Read the model definition and answer for the solid it produces. Units are mm, in the model's axes. A direction names the side the tool comes from. Round coordinates to 2 decimals unless told otherwise and drop trailing zeros. Order: outer loops, then holes, each group sorted by start corner. A loop starts at its lowest first (then second) coordinate and runs counter-clockwise, first axis right, second up.
from build123d import *

# Parameters (mm, degrees)
BOSS_EXTRUDE1_DEPTH  = 10.16
SKETCH2_R            = 2.032
BOSS_EXTRUDE2_DEPTH  = 3.302
SKETCH3_W            = 1.778
SKETCH3_H            = 8.255
BOSS_EXTRUDE3_DEPTH  = 12.7
SKETCH4_W            = 1.524
SKETCH4_H            = 8.255
BOSS_EXTRUDE4_DEPTH  = 2.286
BOSS_EXTRUDE5_DEPTH  = 2.54
BOSS_EXTRUDE6_DEPTH  = 3.556
SKETCH7_W            = 2.032
SKETCH7_H            = 8.255
BOSS_EXTRUDE7_DEPTH  = 2.032
SKETCH8_W            = 1.524
SKETCH8_H            = 8.255
BOSS_EXTRUDE8_DEPTH  = 4.826
SKETCH9_W            = 1.524
SKETCH9_H            = 22.86
BOSS_EXTRUDE9_DEPTH  = 0.254
FILLET2_R            = 0.254
FILLET4_R            = 0.254
FILLET2_OF_MIRROR1_R = 0.254
FILLET4_OF_MIRROR1_R = 0.254
SKETCH10_R           = 3.7084
CUT_EXTRUDE1_DEPTH   = 1.27


with BuildPart() as part:
    # Sketch1 → Boss-Extrude1 (new body)
    with BuildSketch(Plane(origin=(0, 0, 0), x_dir=(1, 0, 0), z_dir=(0, 1, 0))):
        with BuildLine():
            Line((-64.135, 14.859), (64.135, 14.859))
            ThreePointArc((64.135, 14.859), (65.931051224, 14.115051224), (66.675, 12.319))
            Line((66.675, 12.319), (66.675, -12.319))
            ThreePointArc((66.675, -12.319), (65.931051224, -14.115051224), (64.135, -14.859))
            Line((64.135, -14.859), (-64.135, -14.859))
            ThreePointArc((-64.135, -14.859), (-65.931051224, -14.115051224), (-66.675, -12.319))
            Line((-66.675, -12.319), (-66.675, 12.319))
            ThreePointArc((-66.675, 12.319), (-65.931051224, 14.115051224), (-64.135, 14.859))
        make_face()
    extrude(amount=BOSS_EXTRUDE1_DEPTH)

    # Sketch2 → Boss-Extrude2 (add)
    with BuildSketch(Plane.XY.offset(11.557)):
        with BuildLine():
            Line((-10.033, 10.16), (-10.033, 30.48))
            ThreePointArc((-10.033, 30.48), (-10.776948776, 32.276051224), (-12.573, 33.02))
            Line((-12.573, 33.02), (-61.595, 33.02))
            ThreePointArc((-61.595, 33.02), (-65.187102448, 31.532102448), (-66.675, 27.94))
            Line((-66.675, 27.94), (-66.675, 10.16))
            Line((-66.675, 10.16), (-10.033, 10.16))
        make_face()
        with Locations((-61.087, 27.432)):
            Circle(SKETCH2_R, mode=Mode.SUBTRACT)
    boss_extrude2 = extrude(amount=-BOSS_EXTRUDE2_DEPTH)

    # Sketch3 → Boss-Extrude3 (add)
    with BuildSketch(Plane(origin=(0, 10.16, 0), x_dir=(1, 0, 0), z_dir=(0, 1, 0))):
        with Locations((-65.786, -4.1275)):
            Rectangle(SKETCH3_W, SKETCH3_H)
    boss_extrude3 = extrude(amount=BOSS_EXTRUDE3_DEPTH)

    # Sketch4 → Boss-Extrude4 (add)
    with BuildSketch(Plane(origin=(0, 10.16, 0), x_dir=(1, 0, 0), z_dir=(0, 1, 0))):
        with Locations((-53.975, -4.1275)):
            Rectangle(SKETCH4_W, SKETCH4_H)
    boss_extrude4 = extrude(amount=BOSS_EXTRUDE4_DEPTH)

    # Sketch5 → Boss-Extrude5 (add)
    with BuildSketch(Plane(origin=(0, 10.16, 0), x_dir=(1, 0, 0), z_dir=(0, 1, 0))):
        with BuildLine():
            Line((-48.133, 0), (-49.911, 0))
            ThreePointArc((-49.911, 0), (-45.593, -4.318), (-41.275, 0))
            Line((-41.275, 0), (-43.053, 0))
            ThreePointArc((-43.053, 0), (-45.593, -2.54), (-48.133, 0))
        make_face()
    boss_extrude5 = extrude(amount=BOSS_EXTRUDE5_DEPTH)

    # Sketch6 → Boss-Extrude6 (add)
    with BuildSketch(Plane(origin=(0, 10.16, 0), x_dir=(1, 0, 0), z_dir=(0, 1, 0))):
        with BuildLine():
            Line((-33.909, -1.813922821), (-33.909, -3.654423621))
            ThreePointArc((-33.909, -3.654423621), (-35.576423631, -2.155261469), (-36.195, 0))
            Line((-36.195, 0), (-34.671, 0))
            ThreePointArc((-34.671, 0), (-34.472764292, -0.98373777), (-33.909, -1.813922821))
        make_face()
        with BuildLine():
            Line((-30.353, -1.813922821), (-30.353, -3.654423621))
            ThreePointArc((-30.353, -3.654423621), (-28.685576369, -2.155261469), (-28.067, 0))
            Line((-28.067, 0), (-29.591, 0))
            ThreePointArc((-29.591, 0), (-29.789235708, -0.98373777), (-30.353, -1.813922821))
        make_face()
    boss_extrude6 = extrude(amount=BOSS_EXTRUDE6_DEPTH)

    # Sketch7 → Boss-Extrude7 (add)
    with BuildSketch(Plane(origin=(0, 10.16, 0), x_dir=(1, 0, 0), z_dir=(0, 1, 0))):
        with Locations((-23.749, -4.1275)):
            Rectangle(SKETCH7_W, SKETCH7_H)
    boss_extrude7 = extrude(amount=BOSS_EXTRUDE7_DEPTH)

    # Sketch8 → Boss-Extrude8 (add)
    with BuildSketch(Plane(origin=(0, 10.16, 0), x_dir=(1, 0, 0), z_dir=(0, 1, 0))):
        with Locations((-10.795, -4.1275)):
            Rectangle(SKETCH8_W, SKETCH8_H)
    boss_extrude8 = extrude(amount=BOSS_EXTRUDE8_DEPTH)

    # Sketch9 → Boss-Extrude9 (add)
    with BuildSketch(Plane(origin=(0, 0, 8.255), x_dir=(-1, 0, 0), z_dir=(0, 0, -1))):
        with Locations((14.351, 21.59)):
            Rectangle(SKETCH9_W, SKETCH9_H)
    boss_extrude9 = extrude(amount=BOSS_EXTRUDE9_DEPTH)

    # Fillet2
    fillet2_edges = [part.edges().sort_by_distance(p)[0] for p in [
        (-13.589, 21.59, 8.255),
        (-15.113, 21.59, 8.255),
    ]]
    fillet(fillet2_edges, radius=FILLET2_R - 0.0001)  # a hair under: the kernel refuses the full size

    # Fillet4
    fillet4_edges = [part.edges().sort_by_distance(p)[0] for p in [
        (-14.351, 33.02, 8.001),
    ]]
    fillet(fillet4_edges, radius=FILLET4_R - 0.0001)  # a hair under: the kernel refuses the full size

    # Mirror1: Boss-Extrude2, Boss-Extrude3, Boss-Extrude4, Boss-Extrude5, Boss-Extrude6, Boss-Extrude7, Boss-Extrude8, Boss-Extrude9 across plane
    add(boss_extrude2.mirror(Plane.XY))
    add(boss_extrude3.mirror(Plane.XY))
    add(boss_extrude4.mirror(Plane.XY))
    add(boss_extrude5.mirror(Plane.XY))
    add(boss_extrude6.mirror(Plane.XY))
    add(boss_extrude7.mirror(Plane.XY))
    add(boss_extrude8.mirror(Plane.XY))
    add(boss_extrude9.mirror(Plane.XY))

    # Fillet2 of Mirror1
    fillet2_of_mirror1_edges = [part.edges().sort_by_distance(p)[0] for p in [
        (-13.589, 21.59, -8.255),
        (-15.113, 21.59, -8.255),
    ]]
    fillet(fillet2_of_mirror1_edges, radius=FILLET2_OF_MIRROR1_R - 0.0001)  # a hair under: the kernel refuses the full size

    # Fillet4 of Mirror1
    fillet4_of_mirror1_edges = [part.edges().sort_by_distance(p)[0] for p in [
        (-14.351, 33.02, -8.001),
    ]]
    fillet(fillet4_of_mirror1_edges, radius=FILLET4_OF_MIRROR1_R - 0.0001)  # a hair under: the kernel refuses the full size

    # Sketch10 → Cut-Extrude1 (cut)
    with BuildSketch(Plane(origin=(49.657, 0, 0), x_dir=(0, 0, -1), z_dir=(1, 0, 0))):
        with Locations((-4.064, 12.5984)):
            Circle(SKETCH10_R)
    cut_extrude1 = extrude(amount=-CUT_EXTRUDE1_DEPTH, mode=Mode.SUBTRACT)

    # Mirror2: Cut-Extrude1 across plane
    add(cut_extrude1.mirror(Plane.XY), mode=Mode.SUBTRACT)


solid = part.part
Q1. A cutting plane is placed at B-B, the plane x = -21. Give the vertices of the cut face in (y, z) (3 decimals).
Outcome:
outline: (0, -14.859) - (10.16, -14.859) - (10.16, -11.557) - (33.02, -11.557) - (33.02, -8.255) - (10.16, -8.255) - (10.16, 8.255) - (33.02, 8.255) - (33.02, 11.557) - (10.16, 11.557) - (10.16, 14.859) - (0, 14.859) - close
Q2. A cutting plane is placed at C-C, the plane x = 19. Give the vertices of the cut face in (y, z), plus the area to 3 significant figures.
Outcome:
outline: (0, -14.86) - (10.16, -14.86) - (10.16, 14.86) - (0, 14.86) - close
area: 302 mm2
Q3. For a pull along Z with two mould halves and no side action, classify faces 1 (the face through (16, 10.16, 0)), 2 (the face through (-35, 13.716, 0)), 3 (the face through (-1, 5, -14.859)) as released by +Z, released by -Z, zero draft, split by the parting line, or undercut.
Outcome:
face 1: zero draft
face 2: undercut
face 3: released by -Z
Q4. For faces 4 (the face through (-65.15, 31.57, -9.93)), 5 (the face through (-60, 10.16, 0)), 6 (the face through (-39, 22, -11.557)), determine the directions among +Z, -Z, +X, -X, +Y, -Y from which every point of the face is accessible in a straight line to the end or side of a thin tool.
Outcome:
face 4: +Z, -Z, -X, +Y
face 5: +Y
face 6: -Z, +X, -X, +Y
Q5. Flat-ended cylindrical pins translate along their axes: pin 1 (4 mm diameter, centred on y = 25.5, z = -2.5, fed in from +X); pin 2 (8 mm diameter, centred on x = 25, z = 5.5, fed in from +Y); pin 3 (18.5 mm diameter, centred on x = -46.5, y = 16.5, fed in from -Z); pin 4 (10 mm diameter, centred on y = 17.5, z = 0, fed in from +X). Find the tip coordinate at first contact, or state that the pin passes through.
Outcome:
pin 1: passes through
pin 2: stops at y = 10.16
pin 3: stops at z = -14.86
pin 4: stops at x = -10.03
Q6. Straight lines are drawn through the part: probe 1 along Z at (x, y) = (-18.5, 13) (3 decimals); probe 2 along Y at (x, z) = (-32, -7.5); probe 3 along X at (y, z) = (19.5, 3.25) (3 decimals). For each, find the intervals that lie inside material, in ascending order.
Outcome:
probe 1: z = -11.557 to -8.255, 8.255 to 11.557
probe 2: y = 0 to 10.16
probe 3: x = -66.675 to -64.897
